from build123d import *

# Parameters (mm, degrees)
SKETCH_1_R      = 4.1
EXTRUDE_1_DEPTH = 3


with BuildPart() as part:
    # Эскиз1 → Бобышка-Вытянуть1 (new body)
    with BuildSketch(Plane.XZ.offset(-0.99134831)):
        with BuildLine():
            Line((36.958930758, 76.479058001), (-38.898933619, 76.479058001))
            ThreePointArc((-38.898933619, 76.479058001), (-40.046983916, 76.250696599), (-41.020253962, 75.600378345))
            Line((-41.020253962, 75.600378345), (-118.091321774, -1.470689467))
            ThreePointArc((-118.091321774, -1.470689467), (-118.741640028, -2.443959513), (-118.970001431, -3.592009811))
            Line((-118.970001431, -3.592009811), (-118.970001431, -76.520941999))
            ThreePointArc((-118.970001431, -76.520941999), (-118.091321774, -78.642262342), (-115.970001431, -79.520941999))
            Line((-115.970001431, -79.520941999), (114.029998569, -79.520941999))
            ThreePointArc((114.029998569, -79.520941999), (116.151318913, -78.642262342), (117.029998569, -76.520941999))
            Line((117.029998569, -76.520941999), (117.029998569, -3.592009811))
            ThreePointArc((117.029998569, -3.592009811), (116.801637167, -2.443959513), (116.151318913, -1.470689467))
            Line((116.151318913, -1.470689467), (39.080251101, 75.600378345))
            ThreePointArc((39.080251101, 75.600378345), (38.106981055, 76.250696599), (36.958930758, 76.479058001))
        make_face()
        with Locations(Location((99.029998569, -21.520941999, 0), (0, 0, 90))):  # turned: the seam where the file's is
            Circle(SKETCH_1_R, mode=Mode.SUBTRACT)
        with Locations(Location((59.029998569, -21.520941999, 0), (0, 0, 90))):  # turned: the seam where the file's is
            Circle(SKETCH_1_R, mode=Mode.SUBTRACT)
        with Locations(Location((19.029998569, 58.479058001, 0), (0, 0, 90))):  # turned: the seam where the file's is
            Circle(SKETCH_1_R, mode=Mode.SUBTRACT)
        with Locations(Location((19.029998569, 18.479058001, 0), (0, 0, 90))):  # turned: the seam where the file's is
            Circle(SKETCH_1_R, mode=Mode.SUBTRACT)
        with Locations(Location((19.029998569, -21.520941999, 0), (0, 0, 90))):  # turned: the seam where the file's is
            Circle(SKETCH_1_R, mode=Mode.SUBTRACT)
        with Locations(Location((99.029998569, -61.520941999, 0), (0, 0, 90))):  # turned: the seam where the file's is
            Circle(SKETCH_1_R, mode=Mode.SUBTRACT)
        with Locations(Location((59.029998569, -61.520941999, 0), (0, 0, 90))):  # turned: the seam where the file's is
            Circle(SKETCH_1_R, mode=Mode.SUBTRACT)
        with Locations(Location((19.029998569, -61.520941999, 0), (0, 0, 90))):  # turned: the seam where the file's is
            Circle(SKETCH_1_R, mode=Mode.SUBTRACT)
        with Locations(Location((-100.970001431, -21.520941999, 0), (0, 0, 90))):  # turned: the seam where the file's is
            Circle(SKETCH_1_R, mode=Mode.SUBTRACT)
        with Locations(Location((-60.970001431, -21.520941999, 0), (0, 0, 90))):  # turned: the seam where the file's is
            Circle(SKETCH_1_R, mode=Mode.SUBTRACT)
        with Locations(Location((-20.970001431, 58.479058001, 0), (0, 0, 90))):  # turned: the seam where the file's is
            Circle(SKETCH_1_R, mode=Mode.SUBTRACT)
        with Locations(Location((-20.970001431, 18.479058001, 0), (0, 0, 90))):  # turned: the seam where the file's is
            Circle(SKETCH_1_R, mode=Mode.SUBTRACT)
        with Locations(Location((-20.970001431, -21.520941999, 0), (0, 0, 90))):  # turned: the seam where the file's is
            Circle(SKETCH_1_R, mode=Mode.SUBTRACT)
        with Locations(Location((-100.970001431, -61.520941999, 0), (0, 0, 90))):  # turned: the seam where the file's is
            Circle(SKETCH_1_R, mode=Mode.SUBTRACT)
        with Locations(Location((-60.970001431, -61.520941999, 0), (0, 0, 90))):  # turned: the seam where the file's is
            Circle(SKETCH_1_R, mode=Mode.SUBTRACT)
        with Locations(Location((-20.970001431, -61.520941999, 0), (0, 0, 90))):  # turned: the seam where the file's is
            Circle(SKETCH_1_R, mode=Mode.SUBTRACT)
    extrude(amount=-EXTRUDE_1_DEPTH)


solid = part.part
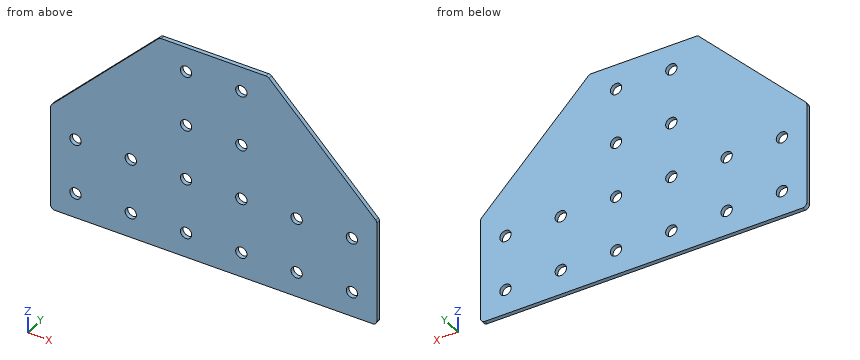
Model file for the job. Use its own axes, mm. Coordinates: 2 decimals unless noted, no trailing zeros. Write each loop counter-clockwise with the first axis right and the second up, starting at its lowest first coordinate (ties: lowest second). Pieces come first, ordered by that corner, then holes. Notation, with made-up numbers: (38.5, -15) -> (65.5, -15) arc R33 cw to (65.5, 22) -> close; hole circle Ø1 at (1, -40). An arc over 180 degrees is marked (long way). One line per item, written item: value. Start each with the question number.
1) Slice it at D-D on x = -74. Write the cut outline in (y, z), then the cut area to 3 significant figures.
2) Slice it at A-A on y = 2.1. Count the separate pieces of the cut face and the enclosed holes in it, then the cut area to 3 significant figures.
3) Slice it at B-B on z = -22.5. Write the cut outline in (x, y), then the cut area to 3 significant figures.
4) Flat gauge pins, fed straight in: pin 1 Ø9.5 at (x, z) = (99.03, -21.52) entering from -Y; pin 2 Ø6.5 at (x, z) = (59.03, -21.52) entering from +Y (3 decimals); pin 3 Ø1.5 at (y, z) = (3, 11.5) entering from -X; pin 4 Ø1 at (x, y) = (-92, 2.5) entering from +Z. Where does each tip first touch, or does it go through?
5) Probe probe 1 along X at (y, z) = (1.95, 18); probe 2 along Z at (x, y) = (20.5, 1.7); probe 3 along Z at (x, y) = (97, 3.55). List the from-to ranges inside material, lowest first.
6) Slice it at C-C on z = 17.5. Write the cut outline in (x, y).
Answers follow:
1. outline: (0.99, -79.52) -> (3.99, -79.52) -> (3.99, 42.62) -> (0.99, 42.62) -> close
1. area: 366 mm2
2. separate pieces: 1
2. enclosed holes: 16
2. area: 29,800 mm2
3. outline: (-118.97, 0.99) -> (-104.95, 0.99) -> (-104.95, 3.99) -> (-118.97, 3.99) -> close; (-96.99, 0.99) -> (-64.95, 0.99) -> (-64.95, 3.99) -> (-96.99, 3.99) -> close; (-56.99, 0.99) -> (-24.95, 0.99) -> (-24.95, 3.99) -> (-56.99, 3.99) -> close; (-16.99, 0.99) -> (15.05, 0.99) -> (15.05, 3.99) -> (-16.99, 3.99) -> close; (23.01, 0.99) -> (55.05, 0.99) -> (55.05, 3.99) -> (23.01, 3.99) -> close; (63.01, 0.99) -> (95.05, 0.99) -> (95.05, 3.99) -> (63.01, 3.99) -> close; (103.01, 0.99) -> (117.03, 0.99) -> (117.03, 3.99) -> (103.01, 3.99) -> close
3. area: 565 mm2
4. pin 1: y = 0.99
4. pin 2: through
4. pin 3: x = -105.87
4. pin 4: z = 25.12
5. probe 1: -98.62 to -25.04, -16.9 to 14.96, 23.1 to 96.68
5. probe 2: -79.52 to -65.35, -57.69 to -25.35, -17.69 to 14.65, 22.31 to 54.65, 62.31 to 76.48
5. probe 3: -79.52 to -65.08, -57.96 to -25.08, -17.96 to 17.68
6. outline: (-99.12, 0.99) -> (-24.95, 0.99) -> (-24.95, 3.99) -> (-99.12, 3.99) -> close; (-16.99, 0.99) -> (15.05, 0.99) -> (15.05, 3.99) -> (-16.99, 3.99) -> close; (23.01, 0.99) -> (97.18, 0.99) -> (97.18, 3.99) -> (23.01, 3.99) -> close
